Input: part model. Units: mm. Frame: model coordinates. A direction names the side the tool comes from. Coordinates: 2 decimals unless noted, no trailing zeros. Write each loop counter-clockwise with the first axis right and the second up, starting at its lowest first coordinate (ties: lowest second). Pieces come first, ordered by that corner, then holes. Notation, with made-up numbers: (19.25, -25) - (36.25, -25) arc R29 cw to (36.25, 14) - close; hole circle Ø10 at (-32.5, -25). An arc over 180 degrees is marked (long way). One line per question, with ' | ' between items. Start each with the question number.
1) First-contact query: P1, Ø2.5, axis at x = 95, y = 16, coming from the -Z side; P2, Ø1, axis at x = 23.5, y = 5.5, coming from the -Z side; P3, Ø0.9, axis at y = 16.5, z = -73, coming from the +X side. Flat tips, straight axial feed; report the tip coordinate or a pass-through.
2) Draft query along X for faces 6 (the flat face through (93.8, 16, 65)), 7 (the cylindrical face through (69.63, 1.67, 53.18)), 8 (the flat face through (-89, 16, -73.8)), 9 (the flat face through (-96.8, 16, -66)). Return one class per face: released by +X, released by -X, zero draft, split by the parting line, or undercut.
3) Section query B-B on z = 0. Return loops of the section in (x, y), and give its area (3 significant figures).
4) Reachability of faces 1 (the cylindrical face through (58.363, 5.07, 51.774)), 2 (the flat face through (47, 5, 44.594)), 3 (the cylindrical face through (-15.625, 5.07, -76.504)), 4 (the cylindrical face through (31.5, 4.93, 17.84)), 5 (the flat face through (15.08, 5, -88)) from +Z, -Z, +X, -X, +Y, -Y: full face, straight path, thin tool, end or side. Return the list, or none.
5) Line query: line 1 (Z direction, x = 0, y = 10.5); line 2 (Z direction, x = 21.5, y = 1.25); line 3 (X direction, y = 16, z = 69.5). Output: solid intervals per line, ascending.
6) Section query A-A on x = 0. Return loops of the section in (y, z).
```python
from build123d import *

# Parameters (mm, degrees)
SKETCH1_R           = 30
BOSS_EXTRUDE1_DEPTH = 10
CUT_EXTRUDE1_START  = -106.930254038
SKETCH2_R           = 1.5
CUT_EXTRUDE1_DEPTH  = 183.700508076
CIRPATTERN1_COUNT   = 3
CIRPATTERN1_ANGLE   = 240
FILLET1_R           = 7
SKETCH4_R           = 30
BOSS_EXTRUDE4_DEPTH = 4
BOSS_EXTRUDE5_DEPTH = 5
FILLET4_R           = 5


with BuildPart() as part:
    # Sketch1 → Boss-Extrude1 (new body)
    with BuildSketch(Plane(origin=(0, 0, 0), x_dir=(1, 0, 0), z_dir=(0, 1, 0))):
        with BuildLine():
            Line((-15.08, 76.19839519), (-15.08, 96.19839519))
            Line((-15.08, 96.19839519), (-7.5, 96.19839519))
            Line((-7.5, 96.19839519), (-7.5, 76.19839519))
            Line((-7.5, 76.19839519), (-23.810275834, 47.948168761))
            ThreePointArc((-23.810275834, 47.948168761), (0, 36.19839519), (23.810275834, 47.948168761))
            Line((23.810275834, 47.948168761), (7.5, 76.19839519))
            Line((7.5, 76.19839519), (7.5, 96.19839519))
            Line((7.5, 96.19839519), (15.08, 96.19839519))
            Line((15.08, 96.19839519), (15.08, 76.19839519))
            ThreePointArc((15.08, 76.19839519), (51.866600724, 29.94519589), (73.529745962, -25.039534506))
            Line((73.529745962, -25.039534506), (90.850254038, -35.039534506))
            Line((90.850254038, -35.039534506), (87.060254038, -41.604007067))
            Line((87.060254038, -41.604007067), (69.739745962, -31.604007067))
            Line((69.739745962, -31.604007067), (53.429470128, -3.353780637))
            ThreePointArc((53.429470128, -3.353780637), (31.348729811, -18.099197595), (29.619194295, -44.594388123))
            Line((29.619194295, -44.594388123), (62.239745962, -44.594388123))
            Line((62.239745962, -44.594388123), (79.560254038, -54.594388123))
            Line((79.560254038, -54.594388123), (75.770254038, -61.158860684))
            Line((75.770254038, -61.158860684), (58.449745962, -51.158860684))
            ThreePointArc((58.449745962, -51.158860684), (0, -59.89039178), (-58.449745962, -51.158860684))
            Line((-58.449745962, -51.158860684), (-75.770254038, -61.158860684))
            Line((-75.770254038, -61.158860684), (-79.560254038, -54.594388123))
            Line((-79.560254038, -54.594388123), (-62.239745962, -44.594388123))
            Line((-62.239745962, -44.594388123), (-29.619194295, -44.594388123))
            ThreePointArc((-29.619194295, -44.594388123), (-31.348729811, -18.099197595), (-53.429470128, -3.353780637))
            Line((-53.429470128, -3.353780637), (-69.739745962, -31.604007067))
            Line((-69.739745962, -31.604007067), (-87.060254038, -41.604007067))
            Line((-87.060254038, -41.604007067), (-90.850254038, -35.039534506))
            Line((-90.850254038, -35.039534506), (-73.529745962, -25.039534506))
            ThreePointArc((-73.529745962, -25.039534506), (-51.866600724, 29.94519589), (-15.08, 76.19839519))
        make_face()
        Circle(SKETCH1_R, mode=Mode.SUBTRACT)
    extrude(amount=BOSS_EXTRUDE1_DEPTH)

    # Sketch2 → Cut-Extrude1 (cut)
    with BuildSketch(Plane(origin=(15.08, 0, 0), x_dir=(0, 0, -1), z_dir=(1, 0, 0)).offset(CUT_EXTRUDE1_START)):
        with Locations((86.19839519, 3)):
            Circle(SKETCH2_R)
    cut_extrude1 = extrude(amount=CUT_EXTRUDE1_DEPTH, mode=Mode.SUBTRACT)

    # CirPattern1: Cut-Extrude1 ×3 about axis
    cirpattern1_axis = Axis((0, 10, 0), (0, -1, 0))
    for i in range(1, CIRPATTERN1_COUNT):
        add(cut_extrude1.rotate(cirpattern1_axis, i * CIRPATTERN1_ANGLE / (CIRPATTERN1_COUNT - 1)), mode=Mode.SUBTRACT)

    # Fillet1
    fillet1_edges = [part.edges().sort_by_distance(p)[0] for p in [
        (-69.739745962, 5, 31.604007067),
        (-73.529745962, 5, 25.039534506),
        (-15.08, 5, -76.19839519),
        (-7.5, 5, -76.19839519),
        (-23.810275834, 5, -47.948168761),
        (23.810275834, 5, -47.948168761),
        (7.5, 5, -76.19839519),
        (15.08, 5, -76.19839519),
        (73.529745962, 5, 25.039534506),
        (69.739745962, 5, 31.604007067),
        (53.429470128, 5, 3.353780637),
        (29.619194295, 5, 44.594388123),
        (62.239745962, 5, 44.594388123),
        (58.449745962, 5, 51.158860684),
        (-58.449745962, 5, 51.158860684),
        (-62.239745962, 5, 44.594388123),
        (-29.619194295, 5, 44.594388123),
        (-53.429470128, 5, 3.353780637),
    ]]
    fillet(fillet1_edges, radius=FILLET1_R)

    # Sketch4 → Boss-Extrude4 (add)
    with BuildSketch(Plane(origin=(0, 10, 0), x_dir=(1, 0, 0), z_dir=(0, 1, 0))):
        with BuildLine():
            Line((-95, -77), (95, -77))
            ThreePointArc((95, -77), (98.535533906, -75.535533906), (100, -72))
            Line((100, -72), (100, 72))
            ThreePointArc((100, 72), (98.535533906, 75.535533906), (95, 77))
            Line((95, 77), (-95, 77))
            ThreePointArc((-95, 77), (-98.535533906, 75.535533906), (-100, 72))
            Line((-100, 72), (-100, -72))
            ThreePointArc((-100, -72), (-98.535533906, -75.535533906), (-95, -77))
        make_face()
        Circle(SKETCH4_R, mode=Mode.SUBTRACT)
        with BuildLine():
            Line((-22.5, 77), (22.5, 77))
            Line((22.5, 77), (22.5, 91.19839519))
            ThreePointArc((22.5, 91.19839519), (21.035533906, 94.733929096), (17.5, 96.19839519))
            Line((17.5, 96.19839519), (-17.5, 96.19839519))
            ThreePointArc((-17.5, 96.19839519), (-21.035533906, 94.733929096), (-22.5, 91.19839519))
            Line((-22.5, 91.19839519), (-22.5, 77))
        make_face()
    extrude(amount=BOSS_EXTRUDE4_DEPTH)

    # Sketch5 → Boss-Extrude5 (add)
    with BuildSketch(Plane(origin=(0, 14, 0), x_dir=(1, 0, 0), z_dir=(0, 1, 0))):
        Polygon((-96.8, 73.8), (-81.8, 73.8), (-81.8, 70.8), (-93.8, 70.8), (-93.8, 58.8), (-96.8, 58.8), align=None)
        Polygon((93.8, 70.8), (81.8, 70.8), (81.8, 73.8), (96.8, 73.8), (96.8, 58.8), (93.8, 58.8), align=None)
        Polygon((93.8, -58.8), (93.8, -70.8), (81.8, -70.8), (81.8, -73.8), (96.8, -73.8), (96.8, -58.8), align=None)
        Polygon((-93.8, -58.8), (-96.8, -58.8), (-96.8, -73.8), (-81.8, -73.8), (-81.8, -70.8), (-93.8, -70.8), align=None)
    extrude(amount=BOSS_EXTRUDE5_DEPTH)

    # Fillet4
    fillet4_edges = [part.edges().sort_by_distance(p)[0] for p in [
        (-22.5, 12, -77),
        (22.5, 12, -77),
    ]]
    fillet(fillet4_edges, radius=FILLET4_R)


solid = part.part
```
Answer key:
1) P1: z = -73.8 | P2: z = -68.39 | P3: x = 96.8
2) face 6: undercut | face 7: undercut | face 8: zero draft | face 9: released by -X
3) outline: (-100, 10) - (-65.99, 10) - (-65.99, 0) - (-30, 0) - (-30, 14) - (-100, 14) - close; (30, 0) - (65.99, 0) - (65.99, 10) - (100, 10) - (100, 14) - (30, 14) - close | area: 1,280 mm²
4) face 1: +Z, -Y | face 2: +X, -Y | face 3: -Z, -X, -Y | face 4: -Y | face 5: -Z, +X, -Y
5) line 1: -96.2 to -30, 30 to 77 | line 2: -69.94 to -51.9, -45.92 to -20.92, 20.92 to 58.73 | line 3: -96.8 to -93.8, 93.8 to 96.8
6) outline: (0, -36.2) - (10, -36.2) - (10, -96.2) - (14, -96.2) - (14, -30) - (0, -30) - close; (0, 30) - (14, 30) - (14, 77) - (10, 77) - (10, 59.89) - (0, 59.89) - close
